```python
from build123d import *

# Parameters (mm, degrees)
SKETCH1_R             = 2.54
SKETCH1_R_2           = 1.7907
BOSS_EXTRUDE1_DEPTH   = 2.3876
BOSS_EXTRUDE1_2_DEPTH = 2.3876
SKETCH3_R             = 1.7907
BOSS_EXTRUDE2_DEPTH   = 1.2446


with BuildPart() as part:
    # Sketch1 → Boss-Extrude1 (new body, symmetric)
    with BuildSketch(Plane.XY):
        with Locations((-4.7625, 0)):
            Circle(SKETCH1_R)
        with Locations((-4.7625, 0)):
            Circle(SKETCH1_R_2, mode=Mode.SUBTRACT)
    extrude(amount=BOSS_EXTRUDE1_DEPTH, both=True)



with BuildPart() as body_2:
    # Sketch1 → Boss-Extrude1 2 (new body, symmetric)
    with BuildSketch(Plane.XY):
        with Locations((4.7625, 0)):
            Circle(SKETCH1_R)
        with Locations((4.7625, 0)):
            Circle(SKETCH1_R_2, mode=Mode.SUBTRACT)
    extrude(amount=BOSS_EXTRUDE1_2_DEPTH, both=True)


with BuildPart() as part_1:
    add(part.part)

    add(body_2.part)  # Boss-Extrude2 merges body 2
    # Sketch3 → Boss-Extrude2 (add)
    with BuildSketch(Plane.XY.offset(2.3876)):
        with BuildLine():
            ThreePointArc((-2.38125, 3.813379876), (-9.2583, 0), (-2.38125, -3.813379876))
            ThreePointArc((-2.38125, -3.813379876), (0, -3.130959752), (2.38125, -3.813379876))
            ThreePointArc((2.38125, -3.813379876), (9.2583, 0), (2.38125, 3.813379876))
            ThreePointArc((2.38125, 3.813379876), (0, 3.130959752), (-2.38125, 3.813379876))
        make_face()
        with Locations((-4.7625, 0)):
            Circle(SKETCH3_R, mode=Mode.SUBTRACT)
        with Locations((4.7625, 0)):
            Circle(SKETCH3_R, mode=Mode.SUBTRACT)
    boss_extrude2 = extrude(amount=BOSS_EXTRUDE2_DEPTH)

    # Mirror3: Boss-Extrude2 across plane
    add(boss_extrude2.mirror(Plane.XY))


solid = part_1.part
```
CAD build for the part. Positions are in the model's coordinates, mm. A direction names the side the tool comes from. Coordinates: 2 decimals unless noted, no trailing zeros. Order: outer loops, then holes, each group sorted by start corner. A loop starts at its lowest first (then second) coordinate and runs counter-clockwise, first axis right, second up. Notation, with made-up numbers: M 55.5,2 L 95.5,2 A25 cw 95.5,37 Z; hole C 25,-9 d9. An arc over 180 degrees is marked long. Write each question's results on one line, items separated by ' | '. Start each with the question number.
Q1. Cut at A-A (y = 0). List the corners of the cut face in (x, z).
Q2. Cut at D-D (y = 2). List the corners of the cut face in (x, z), then the cut area to 3 significant figures.
Q3. Cut at B-B (z = 1.5). List the corners of the cut face in (x, y).
Q4. Cut at C-C (x = -4.25). List the corners of the cut face in (y, z).
Q5. Flat gauge pins, fed straight in: P1, Ø2, axis at y = 0, z = -0.5, coming from the +X side; P2, Ø1, axis at y = 3, z = 2.5, coming from the +X side. Where does each tip first touch, or does it go through?
Q6. Drill centre lines: probe 1 along Z at (x, y) = (2, 1); probe 2 along X at (y, z) = (1.5, 0.25); probe 3 along X at (y, z) = (0.75, 0.25). Where is each one in solid material? Low to high. Write a range as from..to.
Q7. Pull direction Z, two halves, no side cores. Call faces 3 (the cylindrical face through (-3.054, 0.538, 0.051)), 4 (the flat face through (0, 0, -2.388)), 5 (the flat face through (0, 0, -3.632)), 6 (the flat face through (0, 0, 3.632)): +Z half, -Z half, draft (parallel to the pull), parting line (faces both ways), or undercut.
Q8. Which spindle directions (+Z, -Z, +X, -X, +Y, -Y) get a long thin tool onto all of the face, cutting with end or side? Do faces 1 (the flat face through (0, 0, 2.388)), 2 (the cylindrical face through (2.974, 0.079, 0.051)). Say none if no direction does.
Found:
1) outline: M -9.26,-3.63 L -6.55,-3.63 L -6.55,3.63 L -9.26,3.63 L -9.26,2.39 L -7.3,2.39 L -7.3,-2.39 L -9.26,-2.39 Z; M -2.97,-3.63 L 2.97,-3.63 L 2.97,3.63 L -2.97,3.63 Z; M 6.55,-3.63 L 9.26,-3.63 L 9.26,-2.39 L 7.3,-2.39 L 7.3,2.39 L 9.26,2.39 L 9.26,3.63 L 6.55,3.63 Z; hole M -2.22,-2.39 L 2.22,-2.39 L 2.22,2.39 L -2.22,2.39 Z
2) outline: M -8.79,-3.63 L 8.79,-3.63 L 8.79,-2.39 L 6.33,-2.39 L 6.33,2.39 L 8.79,2.39 L 8.79,3.63 L -8.79,3.63 L -8.79,2.39 L -6.33,2.39 L -6.33,-2.39 L -8.79,-2.39 Z; hole M -3.2,-2.39 L 3.2,-2.39 L 3.2,2.39 L -3.2,2.39 Z | area: 73.7 mm²
3) outline: C -4.76,0 d5.08; C 4.76,0 d5.08; hole C -4.76,0 d3.58; hole C 4.76,0 d3.58
4) outline: M -4.47,-3.63 L -1.72,-3.63 L -1.72,3.63 L -4.47,3.63 L -4.47,2.39 L -2.49,2.39 L -2.49,-2.39 L -4.47,-2.39 Z; M 1.72,-3.63 L 4.47,-3.63 L 4.47,-2.39 L 2.49,-2.39 L 2.49,2.39 L 4.47,2.39 L 4.47,3.63 L 1.72,3.63 Z
5) P1: x = 7.3 | P2: x = 8.5
6) probe 1: -3.63..-2.39, 2.39..3.63 | probe 2: -6.81..-5.74, -3.78..-2.71, 2.71..3.78, 5.74..6.81 | probe 3: -7.19..-6.39, -3.14..-2.34, 2.34..3.14, 6.39..7.19
7) face 3: draft | face 4: undercut | face 5: -Z half | face 6: +Z half
8) face 1: none | face 2: +Z, -Z
